```python
from build123d import *

# Parameters (mm, degrees)
SKETCH1_R           = 0.635
BOSS_EXTRUDE1_DEPTH = 1.6


with BuildPart() as part:
    # Sketch1 → Boss-Extrude1 (new body)
    with BuildSketch(Plane(origin=(0, 0, 0), x_dir=(1, 0, 0), z_dir=(0, 1, 0))):
        Polygon((0, 7.62), (0, -7.62), (-7.62, -7.62), (-7.62, 0), (-7.62, 7.62), align=None)
        with Locations((-6.35, 6.35)):
            Circle(SKETCH1_R, mode=Mode.SUBTRACT)
        with Locations((-6.35, 3.81)):
            Circle(SKETCH1_R, mode=Mode.SUBTRACT)
        with Locations((-6.35, 1.27)):
            Circle(SKETCH1_R, mode=Mode.SUBTRACT)
        with Locations((-6.35, -1.27)):
            Circle(SKETCH1_R, mode=Mode.SUBTRACT)
        with Locations((-6.35, -3.81)):
            Circle(SKETCH1_R, mode=Mode.SUBTRACT)
        with Locations((-6.35, -6.35)):
            Circle(SKETCH1_R, mode=Mode.SUBTRACT)
    boss_extrude1 = extrude(amount=BOSS_EXTRUDE1_DEPTH)

    # Mirror1: Boss-Extrude1 across plane
    add(boss_extrude1.mirror(Plane(origin=(0, 1.6, -7.62), x_dir=(0, 0, 1), z_dir=(-1, 0, 0))))


solid = part.part
```
Read the model definition and answer for the solid it produces. Units are mm, in the model's axes. Coordinates: 2 decimals unless noted, no trailing zeros. Write each loop counter-clockwise with the first axis right and the second up, starting at its lowest first coordinate (ties: lowest second). Pieces come first, ordered by that corner, then holes. Notation, with made-up numbers: (3, -28.5) -> (56, -28.5) arc R16 ccw to (56, 0.5) -> close; hole circle Ø1 at (8, 43.25). An arc over 180 degrees is marked (long way). Write item = value, one per line.
(1) Section A-A on z = -6.35 is taken. Write down the section's boundary in (x, y) (3 decimals), plus the area to 3 significant figures.
From the geometry:
outline = (-7.62, 0) -> (-6.985, 0) -> (-6.985, 1.6) -> (-7.62, 1.6) -> close; (-5.715, 0) -> (5.715, 0) -> (5.715, 1.6) -> (-5.715, 1.6) -> close; (6.985, 0) -> (7.62, 0) -> (7.62, 1.6) -> (6.985, 1.6) -> close
area = 20.3 mm2
(2) Section D-D on z = 1.5 is taken. Write down the section's boundary in (x, y), plus the area to 3 significant figures.
From the geometry:
outline = (-7.62, 0) -> (-6.94, 0) -> (-6.94, 1.6) -> (-7.62, 1.6) -> close; (-5.76, 0) -> (5.76, 0) -> (5.76, 1.6) -> (-5.76, 1.6) -> close; (6.94, 0) -> (7.62, 0) -> (7.62, 1.6) -> (6.94, 1.6) -> close
area = 20.6 mm2
(3) For a pull along Z with two mould halves and no side action, classify faces 1 (the face through (-6.85, 0.79, 4.2)), 2 (the face through (-7.62, 1, 0)), 3 (the face through (0, 1, 7.62)), 4 (the face through (0, 1, -7.62)) as +Z half, -Z half, draft (parallel to the pull), parting line (faces both ways), or undercut.
From the geometry:
face_1 = undercut
face_2 = draft
face_3 = +Z half
face_4 = -Z half
(4) Section B-B on x = 6.35 is taken. Write down the section's boundary in (y, z) (3 decimals).
From the geometry:
outline = (0, -7.62) -> (1.6, -7.62) -> (1.6, -6.985) -> (0, -6.985) -> close; (0, -5.715) -> (1.6, -5.715) -> (1.6, -4.445) -> (0, -4.445) -> close; (0, -3.175) -> (1.6, -3.175) -> (1.6, -1.905) -> (0, -1.905) -> close; (0, -0.635) -> (1.6, -0.635) -> (1.6, 0.635) -> (0, 0.635) -> close; (0, 1.905) -> (1.6, 1.905) -> (1.6, 3.175) -> (0, 3.175) -> close; (0, 4.445) -> (1.6, 4.445) -> (1.6, 5.715) -> (0, 5.715) -> close; (0, 6.985) -> (1.6, 6.985) -> (1.6, 7.62) -> (0, 7.62) -> close
(5) Given pin 1 Ø1.1 at (x, z) = (-6.35, -1.27) entering from -Y, flat-ended and moving along its own axis, determine where the tip first touches the part or whether it passes through.
From the geometry:
pin_1 = through
(6) Section C-C on y = 1.15 is taken. Count the separate pieces of the cut face and the enclosed holes in it, plus the area to 3 significant figures.
From the geometry:
separate_pieces = 1
enclosed_holes = 12
area = 217 mm2
(7) Straight lines are drawn through the part: L1, parallel to X at y = 0.3, z = 1; L2, parallel to X at y = 0.75, z = 1.27 (3 decimals). For each, find the intervals that lie inside material, in ascending order. Write a range as from..to.
From the geometry:
L1 = -7.62..-6.92, -5.78..5.78, 6.92..7.62
L2 = -7.62..-6.985, -5.715..5.715, 6.985..7.62
